Verification items for the finished model (mm, model axes). A direction names the side the tool comes from. Give positions to 0.01 mm unless a question says otherwise; leave off trailing zeros. Loops run counter-clockwise (first coordinate to the right, second up) from the corner with the lowest first, then second, coordinate; pieces in that order, holes last. Notation, with made-up numbers: M -16.75,15 L 34.25,15 A27 ccw 34.25,46 Z; hole C 29.25,40 d10. An arc over 180 degrees is marked long. Use CSV: the item, a comma, the result in double quotes.
from build123d import *

# Parameters (mm, degrees)
F0_R     = 5
F0_R_2   = 2.15
F1_DEPTH = 3.5


with BuildPart() as f1:
    # F0 (on Top) → F1 (new body)
    with BuildSketch(Plane.XY):
        Polygon((-2.071068, 5), (-5, 5), (-5, 2.433351), (-7.071068, 0), (-5, -1.708784), (-5, -5), (-2.071068, -5), (0, -7.071068), (2.071068, -5), (5, -5), (5, -2.071068), (7.071068, 0), (5, 2.071068), (5, 5), (2.071068, 5), (0, 7.071068), align=None)
        Circle(F0_R, mode=Mode.SUBTRACT)
        Circle(F0_R)
        Circle(F0_R_2, mode=Mode.SUBTRACT)
    extrude(amount=F1_DEPTH)


solid = f1.part
(1) Mould release check, pull along Y, two halves, no side actions. Record for faces 1 (the flat face through (5, -4, 2)), 2 (the cylindrical face through (-2.15, 0.09, 1.73)), 3 (the flat face through (4, -5, 2)): released by +Y, released by -Y, zero draft, split by the parting line, or undercut.
Calculated:
face 1,"zero draft"
face 2,"undercut"
face 3,"released by -Y"
(2) Section check B-B on x = -1. Record the cut outline in (y, z), plus the area to 3 significant figures.
Calculated:
outline,"M -6.07,0 L -1.9,0 L -1.9,3.5 L -6.07,3.5 Z; M 1.9,0 L 6.07,0 L 6.07,3.5 L 1.9,3.5 Z"
area,"29.2 mm²"
(3) Scan lines: L1, parallel to Y at x = 4, z = 2.2; L2, parallel to Y at x = -1.5, z = 3.3; L3, parallel to Y at x = -1.75, z = 2.5. Record each from-to range of solid material in increasing order. Write a range as from..to.
Calculated:
L1,"y = -5..5"
L2,"y = -5.57..-1.54, 1.54..5.57"
L3,"y = -5.32..-1.25, 1.25..5.32"
(4) Section check C-C on y = 1. Record the cut outline in (x, z), plus the area to 3 significant figures.
Calculated:
outline,"M -6.22,0 L -1.9,0 L -1.9,3.5 L -6.22,3.5 Z; M 1.9,0 L 6.07,0 L 6.07,3.5 L 1.9,3.5 Z"
area,"29.7 mm²"
(5) Section check A-A on z = 3. Record the cut outline in (x, y), plus the area to 3 significant figures.
Calculated:
outline,"M -7.07,0 L -5,-1.71 L -5,-5 L -2.07,-5 L 0,-7.07 L 2.07,-5 L 5,-5 L 5,-2.07 L 7.07,0 L 5,2.07 L 5,5 L 2.07,5 L 0,7.07 L -2.07,5 L -5,5 L -5,2.43 Z; hole C 0,0 d4.3"
area,"103 mm²"
(6) Tool access check on faces 4 (the flat face through (5, 4, 2)), 5 (the flat face through (-5, -3, 2)), 6 (the flat face through (-4, 5, 2)). Record the directions out of +Z, -Z, +X, -X, +Y, -Y that give a thin tool (end or side, any length) a straight path to the whole face; none if there is none.
Calculated:
face 4,"+Z, -Z, +X, +Y"
face 5,"+Z, -Z, -X, -Y"
face 6,"+Z, -Z, -X, +Y"
(7) Section check D-D on y = -3. Record the cut outline in (x, z), plus the area to 3 significant figures.
Calculated:
outline,"M -5,0 L 5,0 L 5,3.5 L -5,3.5 Z"
area,"35.0 mm²"
(8) Depth check by flat-ended pin: pin 1 Ø0.9 at (x, z) = (3.5, 1) entering from +Y; pin 2 Ø2 at (y, z) = (0.5, 1.5) entering from -X; pin 3 Ø1.6 at (y, z) = (-3, 1.5) entering from -X. Enter the tip coordinate at first touch or a pass-through.
Calculated:
pin 1,"stops at y = 5"
pin 2,"stops at x = -7.07"
pin 3,"stops at x = -5"
